Verification items for the finished model (mm, model axes). Face numbers are marked on the shaded views. A direction names the side the tool comes from. Coordinates: 2 decimals unless noted, no trailing zeros. Write each loop counter-clockwise with the first axis right and the second up, starting at its lowest first coordinate (ties: lowest second). Pieces come first, ordered by that corner, then holes. Notation, with made-up numbers: (42.5, 60) -> (49.5, 60) arc R17 cw to (49.5, 86) -> close; hole circle Ø2 at (36.5, 3). An arc over 180 degrees is marked (long way). Write item = value, one per line. Start each with the question number.
(1) Mould release check, pull along X, two halves, no side actions. Record for the marked faces 4, 5 and 6: released by +X, released by -X, zero draft, split by the parting line, or undercut.
(2) Section check C-C (y = 39). Record the cut outline in (x, z), plus the area to 3 significant figures.
(3) Section check D-D (x = 0). Record the cut outline in (y, z), plus the area to 3 significant figures.
(4) Section check B-B (y = -57). Record the cut outline in (x, z).
(5) Material ranges on probe 1 along Y at (x, z) = (-36, 21.25); probe 2 along X at (y, z) = (-24, 19), recorded low to high. Write a range as [from, to].
(6) Gauge pin test, flat ends, axial feed: pin 1 Ø1 at (x, y) = (21, -25.5) entering from +Z; pin 2 Ø1 at (y, z) = (-40, 5) entering from -X; pin 3 Ø6 at (y, z) = (27, 11.5) entering from +X. Record the tip position at first contact, or that the pin passes through.
(7) Set-up check for the marked faces 1, 2 and 3: record each of +Z, -Z, +X, -X, +Y, -Y from which the full face is reachable in a straight line by a thin tool's end or side.
(8) Section check A-A (z = 23.25). Record the cut outline in (x, y), plus the area to 3 significant figures.
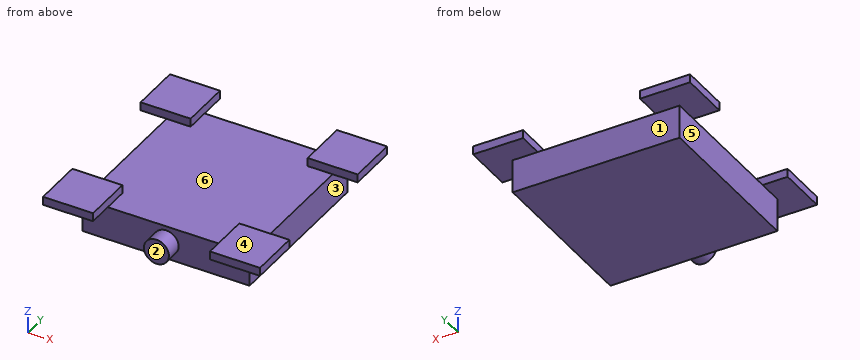
```python
from build123d import *

# Parameters (mm, degrees)
SKETCH_W     = 100
SKETCH_H     = 100
PAD_DEPTH    = 20
SKETCH001_W  = 30
SKETCH001_H  = 30
PAD001_DEPTH = 5
SKETCH002_R  = 7.5
PAD002_DEPTH = 10


with BuildPart() as part:
    # Sketch → Pad (new body)
    with BuildSketch(Plane.XY):
        Rectangle(SKETCH_W, SKETCH_H)
    extrude(amount=PAD_DEPTH)

    # Sketch001 (on Face6 of Pad) → Pad001 (join)
    with BuildSketch(Plane.XY.offset(20)):
        with Locations((-50.543835, 50.845081)):
            Rectangle(SKETCH001_W, SKETCH001_H)
        with Locations((-50, -50)):
            Rectangle(SKETCH001_W, SKETCH001_H)
        with Locations((50, -50)):
            Rectangle(SKETCH001_W, SKETCH001_H)
        with Locations((50, 50)):
            Rectangle(SKETCH001_W, SKETCH001_H)
    extrude(amount=PAD001_DEPTH)

    # Sketch002 (on Face1 of Pad001) → Pad002 (join)
    with BuildSketch(Plane.XZ.offset(50)):
        with Locations((0, 10)):
            Circle(SKETCH002_R)
    extrude(amount=PAD002_DEPTH)


solid = part.part
```
Response:
q1.face_4 = zero draft
q1.face_5 = released by -X
q1.face_6 = undercut
q2.outline = (-65.54, 20) -> (-50, 20) -> (-50, 0) -> (50, 0) -> (50, 20) -> (65, 20) -> (65, 25) -> (35, 25) -> (35, 20) -> (-35.54, 20) -> (-35.54, 25) -> (-65.54, 25) -> close
q2.area = 2,300 mm2
q3.outline = (-60, 2.5) -> (-50, 2.5) -> (-50, 0) -> (50, 0) -> (50, 20) -> (-50, 20) -> (-50, 17.5) -> (-60, 17.5) -> close
q3.area = 2,150 mm2
q4.outline = (-65, 20) -> (-35, 20) -> (-35, 25) -> (-65, 25) -> close; circle Ø15 at (0, 10); (35, 20) -> (65, 20) -> (65, 25) -> (35, 25) -> close
q5.probe_1 = [-65, -35], [35.85, 65.85]
q5.probe_2 = [-50, 50]
q6.pin_1 = 20
q6.pin_2 = -50
q6.pin_3 = 50
q7.face_1 = -Z, +X, -X, +Y
q7.face_2 = +Z, -Z, +X, -X, -Y
q7.face_3 = -Z, +X, +Y, -Y
q8.outline = (-65.54, 35.85) -> (-35.54, 35.85) -> (-35.54, 65.85) -> (-65.54, 65.85) -> close; (-65, -65) -> (-35, -65) -> (-35, -35) -> (-65, -35) -> close; (35, -65) -> (65, -65) -> (65, -35) -> (35, -35) -> close; (35, 35) -> (65, 35) -> (65, 65) -> (35, 65) -> close
q8.area = 3,600 mm2
